Geometry: final body of the model. Coordinates: model frame, mm. A direction names the side the tool comes from. Give positions to 0.01 mm unless a question says otherwise; leave off trailing zeros. Order: outer loops, then holes, each group sorted by start corner. A loop starts at its lowest first (then second) coordinate and runs counter-clockwise, first axis right, second up. Notation, with made-up numbers: (31.25, 80) - (86.25, 80) arc R29 cw to (86.25, 112) - close; hole circle Ø5 at (-4, 68). An arc over 180 degrees is marked (long way). Put each result on its own line as item: value. Start each with the question number.
1. Section B-B on y = 63.5. Return the cut outline in (x, z).
2. Section A-A on z = 7. Count the separate pieces of the cut face and the enclosed holes in it, plus the area to 3 significant figures.
3. Set-up query: faces 1 (the cylindrical face through (17.5, 63.6, 7.1)), 2 (the flat face through (-46.1, 10, 4.6)), 3 (the flat face through (25, 66, 7)), 4 (the flat face through (0, 77.5, 7)), 5 (the flat face through (-25, 66, 7)). Return all of +Z, -Z, +X, -X, +Y, -Y with unobstructed straight access to the full face (end or side cutting, diameter ignored); none if empty.
4. Mould query, pull axis Z, two halves, no side actions, for faces 6 (the cylindrical face through (-38.23, 18.49, 6.78)), 7 (the cylindrical face through (-23.797, 76.359, 6.902)), 8 (the flat face through (-1, 48, 0)). Classes: pulls with the +Z half, pulls with the -Z half, needs draft (parallel to the pull), parting line crosses it, or undercut.
5. Section C-C on y = 17. Return the cut outline in (x, z), plus the area to 3 significant figures.
6. First-contact query: P1, Ø8, axis at x = -21, z = 3, coming from the -Y side; P2, Ø8, axis at y = 33.5, z = 3.5, coming from the +X side; P3, Ø1.5, axis at y = 24.5, z = 1.5, coming from the -X side. Flat tips, straight axial feed; report the tip coordinate or a pass-through.
7. Section D-D on x = 42. Return the cut outline in (y, z).
8. Ray query, line 1 along Y through (x, z) = (-1, 10.5); line 2 along Y through (x, z) = (-20, 7); line 3 along Y through (x, z) = (-21.5, 12.25). Return the intervals inside material, ascending. Write a range as from..to.
from build123d import *

# Parameters (mm, degrees)
F0_R      = 50
F0_R_2    = 37.5
F1_DEPTH  = 14
F2_W      = 110
F2_H      = 64.89666
F3_DEPTH  = 14.001
F4_R      = 3
F5_DEPTH  = 50.001
F7_R      = 5.5
F8_DEPTH  = 25
F10_DEPTH = 14
F11_R     = 2.5
F12_DEPTH = 14.001


with BuildPart() as f1:
    # F0 (on Top) → F1 (new body)
    with BuildSketch(Plane.XY):
        Circle(F0_R)
        Circle(F0_R_2, mode=Mode.SUBTRACT)
    extrude(amount=F1_DEPTH)

    # F2 (on face) → F3 (cut, through all)
    with BuildSketch(Plane.XY.offset(14)):
        with Locations((0, -30.94833)):
            Rectangle(F2_W, F2_H)
    extrude(amount=-F3_DEPTH, mode=Mode.SUBTRACT)

    # F4 (on Front) → F5 (cut, through all)
    with BuildSketch(Plane.XZ):
        with Locations((-43.723741, 7)):
            Circle(F4_R)
        with Locations((43.723741, 7)):
            Circle(F4_R)
    extrude(amount=-F5_DEPTH, mode=Mode.SUBTRACT)

    # F7 (on offset) → F8 (cut)
    with BuildSketch(Plane.XZ.offset(-10)):
        with Locations((43.723741, 7)):
            Circle(F7_R)
        with Locations((-43.723741, 7)):
            Circle(F7_R)
    extrude(amount=-F8_DEPTH, mode=Mode.SUBTRACT)

    # F9 (on Top) → F10 (join, through all)
    with BuildSketch(Plane.XY):
        with BuildLine():
            ThreePointArc((25, 73.5), (23.828427, 76.328427), (21, 77.5))
            Line((21, 77.5), (-21, 77.5))
            ThreePointArc((-21, 77.5), (-23.828427, 76.328427), (-25, 73.5))
            Line((-25, 73.5), (-25, 58.320619))
            ThreePointArc((-25, 58.320619), (-27.088522, 47.322921), (-33.063292, 37.856484))
            Line((-33.063292, 37.856484), (-36.56118, 34.106892))
            Line((-36.56118, 34.106892), (0, 41.856416))
            Line((0, 41.856416), (36.56118, 34.106892))
            Line((36.56118, 34.106892), (33.063292, 37.856484))
            ThreePointArc((33.063292, 37.856484), (27.088522, 47.322921), (25, 58.320619))
            Line((25, 58.320619), (25, 73.5))
        make_face()
    extrude(amount=F10_DEPTH)

    # F11 (on face) → F12 (cut, through all)
    with BuildSketch(Plane.XY.offset(14)):
        with Locations((-20, 63.5)):
            Circle(F11_R)
        with Locations((20, 63.5)):
            Circle(F11_R)
    extrude(amount=-F12_DEPTH, mode=Mode.SUBTRACT)


solid = f1.part
Resolved:
1. outline: (-25, 0) - (-22.5, 0) - (-22.5, 14) - (-25, 14) - close; (-17.5, 0) - (17.5, 0) - (17.5, 14) - (-17.5, 14) - close; (22.5, 0) - (25, 0) - (25, 14) - (22.5, 14) - close
2. separate pieces: 3
2. enclosed holes: 2
2. area: 2,790 mm^2
3. face 1: +Z, -Z
3. face 2: +Y
3. face 3: +Z, -Z, +X, +Y
3. face 4: +Z, -Z, +X, -X, +Y
3. face 5: +Z, -Z, -X, +Y
4. face 6: undercut
4. face 7: needs draft
4. face 8: pulls with the -Z half
5. outline: (-47.02, 0) - (-33.43, 0) - (-33.43, 14) - (-47.02, 14) - (-47.02, 11.4) arc R5.5 cw (long way) to (-47.02, 2.6) - close; (33.43, 0) - (47.02, 0) - (47.02, 2.6) arc R5.5 cw (long way) to (47.02, 11.4) - (47.02, 14) - (33.43, 14) - close
5. area: 218 mm^2
6. P1: y = 27.95
6. P2: x = 40.31
6. P3: x = -44
7. outline: (1.5, 0) - (27.13, 0) - (27.13, 1.78) - (10, 1.78) - (10, 4.54) - (1.5, 4.54) - close; (1.5, 9.46) - (10, 9.46) - (10, 12.22) - (27.13, 12.22) - (27.13, 14) - (1.5, 14) - close
8. line 1: 37.49..77.5
8. line 2: 31.72..61, 66..77.5
8. line 3: 30.72..61.5, 65.5..77.47
